from build123d import *

# Parameters (mm, degrees)
SKETCH1_R           = 7.00000696
BOSS_EXTRUDE1_DEPTH = 24
SKETCH2_W           = 9
SKETCH2_H           = 24
CUT_EXTRUDE1_DEPTH  = 32
SKETCH3_OUTSIDE_W   = 45.612
SKETCH3_OUTSIDE_H   = 45.612
CUT_EXTRUDE3_DEPTH  = 68
SKETCH4_R           = 9
CUT_EXTRUDE4_DEPTH  = 67


with BuildPart() as part:
    # Sketch1 → Boss-Extrude1 (new body)
    with BuildSketch(Plane.XY):
        with BuildLine():
            Line((-50.044390832, 27.503498209), (29.955609168, 27.503498209))
            ThreePointArc((29.955609168, 27.503498209), (38.440890542, 7.018216834), (17.955609168, 15.503498209))
            Line((17.955609168, 15.503498209), (17.955609168, 6.136182916))
            Line((17.955609168, 6.136182916), (-39.544390832, 6.003498209))
            Line((-39.544390832, 6.003498209), (-39.544390832, 5.015222645))
            Line((-39.544390832, 5.015222645), (-48.572054411, 5.015222645))
            Line((-48.572054411, 5.015222645), (-48.572054411, 6.003498173))
            Line((-48.572054411, 6.003498173), (-50.044390832, 6.003498173))
            Line((-50.044390832, 6.003498173), (-50.044390832, 27.503498209))
        make_face()
        with Locations((29.955609168, 15.503498209)):
            Circle(SKETCH1_R, mode=Mode.SUBTRACT)
    extrude(amount=BOSS_EXTRUDE1_DEPTH)

    # Sketch2 → Cut-Extrude1 (cut)
    with BuildSketch(Plane(origin=(50, 0, 0), x_dir=(0, 0, -1), z_dir=(1, 0, 0))):
        with Locations((-12.486255169, 15.503498209)):
            Rectangle(SKETCH2_W, SKETCH2_H)
    extrude(amount=-CUT_EXTRUDE1_DEPTH, mode=Mode.SUBTRACT)

    # Sketch3 outside → Cut-Extrude3 (cut)
    with BuildSketch(Plane.ZY.offset(50.044390832)):
        with Locations((12, 15.503)):
            Rectangle(SKETCH3_OUTSIDE_W, SKETCH3_OUTSIDE_H)
        with BuildLine():
            Line((0, 27.503498209), (24, 27.503498209))
            Line((24, 27.503498209), (24, 19.503498209))
            ThreePointArc((24, 19.503498209), (20.795941553, 10.268216816), (12, 6.003498173))
            ThreePointArc((12, 6.003498173), (3.204058447, 10.268216816), (0, 19.503498209))
            Line((0, 19.503498209), (0, 27.503498209))
        make_face(mode=Mode.SUBTRACT)
    extrude(amount=-CUT_EXTRUDE3_DEPTH, mode=Mode.SUBTRACT)

    # Sketch4 → Cut-Extrude4 (cut)
    with BuildSketch(Plane.ZY.offset(50.044390832)):
        with Locations((12, 17.218107651)):
            Circle(SKETCH4_R)
    extrude(amount=-CUT_EXTRUDE4_DEPTH, mode=Mode.SUBTRACT)


solid = part.part
The listing builds one solid part. Answer for the finished solid, in the listing's coordinates (mm). A direction names the side the tool comes from. Coordinates: 2 decimals unless noted, no trailing zeros. Loops run counter-clockwise (first coordinate to the right, second up) from the corner with the lowest first, then second, coordinate; pieces in that order, holes last. Notation, with made-up numbers: (-35, -2.75) -> (24, -2.75) arc R13 cw to (24, 9.25) -> close; hole circle Ø9 at (-12, -26). An arc over 180 degrees is marked (long way). Write item = value, one per line. Start each with the question number.
1) Straight lines are drawn through the part: line 1 (Z direction, x = 21, y = 26.5); line 2 (Y direction, x = -33, z = 12); line 3 (X direction, y = 19, z = 19.25). For each, find the intervals that lie inside material, in ascending order. Write a range as from..to.
2) A tool of negligible diameter and unlimited length cuts with its end or side. For faces 1 (the face through (-16.52, 9.81, 20.37)), 2 (the face through (25, 21, 7.986)), 3 (the face through (17.956, 12, 12)), from which of +Z, -Z, +X, -X, +Y, -Y can it reach the whole face along a straight path? Write none if from no direction.
3) A cutting plane is placed at D-D (z = 16). Give the vertices of the cut face in (x, y), then the cut area to 3 significant figures.
4) A cutting plane is placed at C-C (x = -33). Give the vertices of the cut face in (y, z), then the cut area to 3 significant figures.
5) A cutting plane is placed at A-A (x = 33.5). Give the vertices of the cut face in (y, z).
6) Given pin 1 Ø6 at (x, z) = (5.5, 3.5) entering from -Y; pin 2 Ø1.5 at (x, z) = (6.5, 21.5) entering from -Y; pin 3 Ø5.5 at (y, z) = (13, 12) entering from -X; pin 4 Ø10 at (y, z) = (18.5, 13) entering from +X, each flat-ended and moving along its own axis, determine where each tip first touches the part or whether it passes through.
7) The mould has two halves that part along X. Classify faces 4 (the face through (18, 21, 13)), 5 (the face through (36.63, 17.61, 20.44)), 6 (the face through (-50.044, 25, 17)): released by +X, released by -X, zero draft, split by the parting line, or undercut.
8) A cutting plane is placed at B-B (y = 11.75). Give the vertices of the cut face in (x, z).
Responses:
q1.line_1 = 0..7.99, 16.99..24
q1.line_2 = 6.02..8.22, 26.22..27.5
q1.line_3 = 16.96..23.89, 36.02..41.43
q2.face_1 = +Z, -X, -Y
q2.face_2 = +X, +Y, -Y
q2.face_3 = none
q3.outline = (-50.04, 6.9) -> (17.96, 6.9) -> (17.96, 15.5) arc R12 ccw to (18, 14.47) -> (18, 27.5) -> (-50.04, 27.5) -> (-50.04, 25.28) -> (16.96, 25.28) -> (16.96, 9.16) -> (-50.04, 9.16) -> close
q3.area = 321 mm²
q4.outline = (6.02, 11.78) arc R12.77 ccw to (18, 0) -> (27.5, 0) -> (27.5, 24) -> (18, 24) arc R12.77 ccw to (6.02, 12.22) -> close; hole circle Ø18 at (17.22, 12)
q4.area = 193 mm²
q5.outline = (4.04, 0) -> (9.47, 0) -> (9.47, 7.99) -> (4.04, 7.99) -> close; (4.04, 16.99) -> (9.47, 16.99) -> (9.47, 24) -> (4.04, 24) -> close; (21.54, 0) -> (26.97, 0) -> (26.97, 7.99) -> (21.54, 7.99) -> close; (21.54, 16.99) -> (26.97, 16.99) -> (26.97, 24) -> (21.54, 24) -> close
q6.pin_1 = 7.62
q6.pin_2 = 10.22
q6.pin_3 = 16.96
q6.pin_4 = 41.96
q7.face_4 = released by +X
q7.face_5 = undercut
q7.face_6 = released by -X
q8.outline = (-50.04, 2.07) -> (17.96, 2.07) -> (17.96, 21.93) -> (-50.04, 21.93) -> (-50.04, 19.15) -> (16.96, 19.15) -> (16.96, 4.85) -> (-50.04, 4.85) -> close; (18.56, 0) -> (24.05, 0) -> (24.05, 7.99) -> (18.56, 7.99) -> close; (18.56, 16.99) -> (24.05, 16.99) -> (24.05, 24) -> (18.56, 24) -> close; (35.86, 0) -> (41.35, 0) -> (41.35, 7.99) -> (35.86, 7.99) -> close; (35.86, 16.99) -> (41.35, 16.99) -> (41.35, 24) -> (35.86, 24) -> close
